Can you work these out from the drawing? Everything is in mm from the part's minimum corner. Coordinates: 2 decimals unless noted, no trailing zeros. Loops run counter-clockwise (first coordinate to the right, second up) from the corner with the lowest first, then second, coordinate; pieces in that order, holes last. Notation, with made-up numbers: (55, 4.5) - (81, 4.5) arc R20 cw to (81, 9.5) - close; hole circle Ø6 at (85, 23.25). An arc over 180 degrees is marked (long way). One line per question, with ' | ' between items. Start each with the question number.
1. We'd pull the mould along X, two halves only. Please class the marked faces 1 and 2: pulls with the +X half, pulls with the -X half, needs draft (parallel to the pull), parting line crosses it, or undercut.
2. Please list where these lines run through material, in increasing order: L1, parallel to Y at x = 55, z = 7; L2, parallel to Y at x = 55, z = 2.5; L3, parallel to Z at x = 103, y = 49. Write a range as [from, to].
3. I want a section at C-C, the plane z = 7.25. Write out the boundary of the cut face in (x, y).
4. I want a section at A-A, the plane y = 55. Write out the boundary of the cut face in (x, z), then the cut area to 3 significant figures.
5. I want a section at D-D, the plane z = 1.75. Write out the boundary of the cut face in (x, y).
6. I'm going to push flat-ended pins straight in: P1, Ø16, axis at x = 55, y = 55, coming from the -Z side; P2, Ø4, axis at x = 56, y = 76, coming from the +Z side; P3, Ø5, axis at y = 48, z = 11, coming from the +X side; P4, Ø1, axis at x = 57, z = 8.5, coming from the -Y side. Where does each tip first touch, or does it pass through?
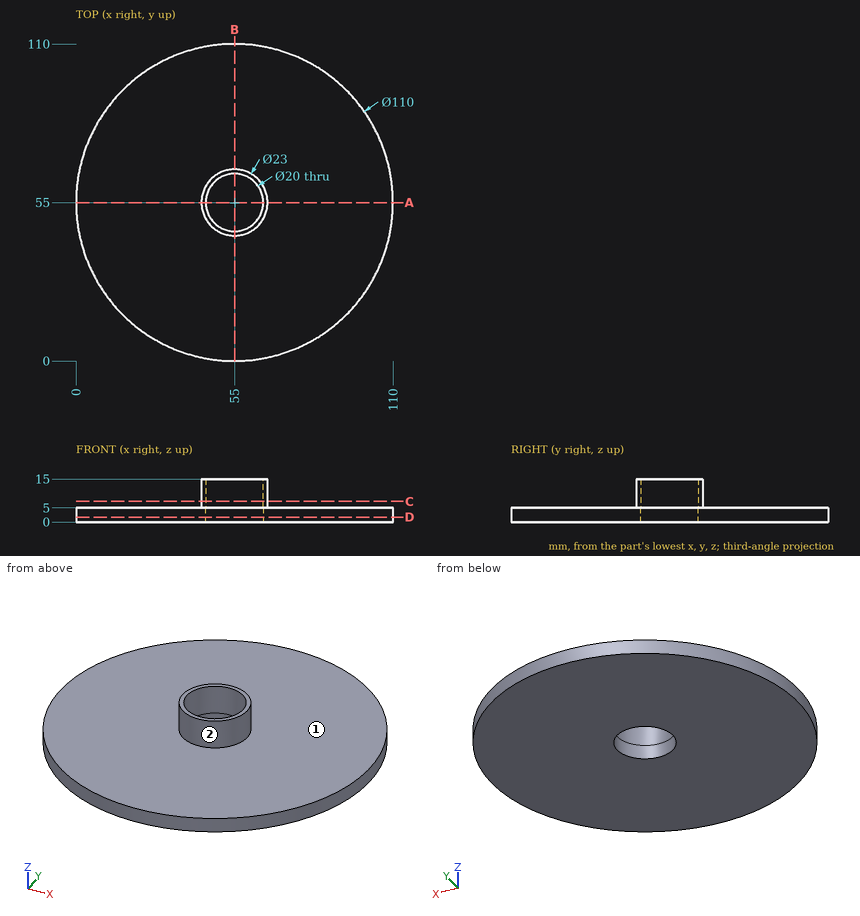
Results are:
1) face 1: needs draft | face 2: parting line crosses it
2) L1: y = [43.5, 45], [65, 66.5] | L2: y = [0, 45], [65, 110] | L3: z = [0, 5]
3) outline: circle Ø23 at (55, 55); hole circle Ø20 at (55, 55)
4) outline: (0, 0) - (45, 0) - (45, 15) - (43.5, 15) - (43.5, 5) - (0, 5) - close; (65, 0) - (110, 0) - (110, 5) - (66.5, 5) - (66.5, 15) - (65, 15) - close | area: 480 mm2
5) outline: circle Ø110 at (55, 55); hole circle Ø20 at (55, 55)
6) P1: passes through | P2: stops at z = 5 | P3: stops at x = 65.58 | P4: stops at y = 43.6
